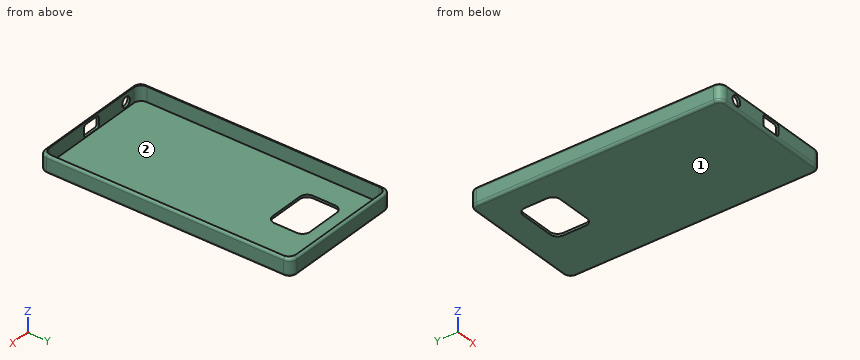
from build123d import *

# Parameters (mm, degrees)
F1_DEPTH = 1
F2_DEPTH = 7
F3_R     = 0.99999
F4_R     = 2
F5_DEPTH = 1


# Not quite as in the source:
# - a fillet or chamfer is up to 0.001 mm smaller than in the source, because OpenCascade refuses the exact size


with BuildPart() as f1:
    # F0 (on Top) → F1 (new body)
    with BuildSketch(Plane.XY):
        with BuildLine():
            Line((26, -48), (26, 48))
            ThreePointArc((26, 48), (25.1213203436, 50.1213203436), (23, 51))
            Line((23, 51), (-23, 51))
            ThreePointArc((-23, 51), (-25.1213203436, 50.1213203436), (-26, 48))
            Line((-26, 48), (-26, -48))
            ThreePointArc((-26, -48), (-25.1213203436, -50.1213203436), (-23, -51))
            Line((-23, -51), (23, -51))
            ThreePointArc((23, -51), (25.1213203436, -50.1213203436), (26, -48))
        make_face()
        with BuildLine():
            ThreePointArc((-25, 47), (-24.1213203436, 49.1213203436), (-22, 50))
            Line((-22, 50), (22, 50))
            ThreePointArc((22, 50), (24.1213203436, 49.1213203436), (25, 47))
            Line((25, 47), (25, -47))
            ThreePointArc((25, -47), (24.1213203436, -49.1213203436), (22, -50))
            Line((22, -50), (-22, -50))
            ThreePointArc((-22, -50), (-24.1213203436, -49.1213203436), (-25, -47))
            Line((-25, -47), (-25, 47))
        make_face(mode=Mode.SUBTRACT)
        with BuildLine():
            Line((22, 50), (-22, 50))
            ThreePointArc((-22, 50), (-24.1213203436, 49.1213203436), (-25, 47))
            Line((-25, 47), (-25, -47))
            ThreePointArc((-25, -47), (-24.1213203436, -49.1213203436), (-22, -50))
            Line((-22, -50), (22, -50))
            ThreePointArc((22, -50), (24.1213203436, -49.1213203436), (25, -47))
            Line((25, -47), (25, 47))
            ThreePointArc((25, 47), (24.1213203436, 49.1213203436), (22, 50))
        make_face()
        with BuildLine():
            ThreePointArc((-15, 37), (-14.1213203436, 39.1213203436), (-12, 40))
            Line((-12, 40), (2, 40))
            ThreePointArc((2, 40), (4.1213203436, 39.1213203436), (5, 37))
            Line((5, 37), (5, 28))
            ThreePointArc((5, 28), (4.1213203436, 25.8786796564), (2, 25))
            Line((2, 25), (-12, 25))
            ThreePointArc((-12, 25), (-14.1213203436, 25.8786796564), (-15, 28))
            Line((-15, 28), (-15, 37))
        make_face(mode=Mode.SUBTRACT)
    extrude(amount=F1_DEPTH)

    # F0 (on Top) → F2 (join)
    with BuildSketch(Plane.XY):
        with BuildLine():
            Line((26, -48), (26, 48))
            ThreePointArc((26, 48), (25.1213203436, 50.1213203436), (23, 51))
            Line((23, 51), (-23, 51))
            ThreePointArc((-23, 51), (-25.1213203436, 50.1213203436), (-26, 48))
            Line((-26, 48), (-26, -48))
            ThreePointArc((-26, -48), (-25.1213203436, -50.1213203436), (-23, -51))
            Line((-23, -51), (23, -51))
            ThreePointArc((23, -51), (25.1213203436, -50.1213203436), (26, -48))
        make_face()
        with BuildLine():
            ThreePointArc((-25, 47), (-24.1213203436, 49.1213203436), (-22, 50))
            Line((-22, 50), (22, 50))
            ThreePointArc((22, 50), (24.1213203436, 49.1213203436), (25, 47))
            Line((25, 47), (25, -47))
            ThreePointArc((25, -47), (24.1213203436, -49.1213203436), (22, -50))
            Line((22, -50), (-22, -50))
            ThreePointArc((-22, -50), (-24.1213203436, -49.1213203436), (-25, -47))
            Line((-25, -47), (-25, 47))
        make_face(mode=Mode.SUBTRACT)
    extrude(amount=F2_DEPTH)

    # F3 (radius 1 in the source; OpenCascade refuses exactly that, so slightly less here)
    f3_edges = [f1.edges().sort_by_distance(p)[0] for p in [
        (26, 0, 0),
        (-26, 0, 7),
    ]]
    fillet(f3_edges, radius=F3_R)

    # F4 (on face) → F5 (cut, through all)
    with BuildSketch(Plane.XZ.offset(51)):
        with BuildLine():
            Line((2.9, 6), (-2.9, 6))
            ThreePointArc((-2.9, 6), (-3.6071067812, 5.7071067812), (-3.9, 5))
            Line((-3.9, 5), (-3.9, 2.2120511904))
            ThreePointArc((-3.9, 2.2120511904), (-3.6071067812, 1.5049444092), (-2.9, 1.2120511904))
            Line((-2.9, 1.2120511904), (2.9, 1.2120511904))
            ThreePointArc((2.9, 1.2120511904), (3.6071067812, 1.5049444092), (3.9, 2.2120511904))
            Line((3.9, 2.2120511904), (3.9, 5))
            ThreePointArc((3.9, 5), (3.6071067812, 5.7071067812), (2.9, 6))
        make_face()
        with Locations((-18, 3.5)):
            Circle(F4_R)
    extrude(amount=-F5_DEPTH, mode=Mode.SUBTRACT)


solid = f1.part
Source: CAD feature listing. Evaluate the final solid. Frame: model axes, mm. Face numbers are marked on the shaded views. Round coordinates to 2 decimals unless told otherwise and drop trailing zeros. Loops run counter-clockwise (first coordinate to the right, second up) from the corner with the lowest first, then second, coordinate; pieces in that order, holes last. Notation, with made-up numbers: M 74.25,23.5 L 109.25,23.5 A23 cw 109.25,61.5 Z; hole C -34.75,76 d5. An arc over 180 degrees is marked long. Answer as CSV lines item,"result".
Q1. Cut plane B-B (z = 3.5). Return the cut outline in (x, y), plus the area to 3 significant figures.
Verdict:
outline,"M -26,-48 A3 ccw -23,-51 L -20,-51 L -20,-50 L -22,-50 A3 cw -25,-47 L -25,47 A3 cw -22,50 L 22,50 A3 cw 25,47 L 25,-47 A3 cw 22,-50 L 3.9,-50 L 3.9,-51 L 23,-51 A3 ccw 26,-48 L 26,48 A3 ccw 23,51 L -23,51 A3 ccw -26,48 Z; M -16,-51 L -3.9,-51 L -3.9,-50 L -16,-50 Z"
area,"292 mm^2"
Q2. Contact query for flat-ended pins moving along their axis: pin 1 (25 mm diameter, centred on x = -4.5, y = 2.5, fed in from +Z); pin 2 (1.8 mm diameter, centred on x = 1.5, z = 3.5, fed in from -Y); pin 3 (0.5 mm diameter, centred on x = 1, y = -50.5, fed in from -Z). Output: stop coordinate, or through.
Verdict:
pin 1,"stops at z = 1"
pin 2,"stops at y = 50"
pin 3,"stops at z = 0.03"
Q3. Line query: line 1 along Y through (x, z) = (-8.5, 2.5); line 2 along X through (y, z) = (-45, 5.5); line 3 along Y through (x, z) = (0.5, 3). Output: solid intervals per line, ascending.
Verdict:
line 1,"y = -51 to -50, 50 to 51"
line 2,"x = -26 to -25, 25 to 26"
line 3,"y = 50 to 51"
Q4. Pull-direction query (X, two-part tool) for the marked faces 1 and 2; classes: +X half, -X half, draft (parallel to the pull), parting line (faces both ways), or undercut.
Verdict:
face 1,"draft"
face 2,"undercut"
Q5. Cut plane D-D (x = 1). Count the separate pieces of the cut face and the enclosed holes in it, plus the area to 3 significant figures.
Verdict:
separate pieces,"3"
enclosed holes,"0"
area,"93.4 mm^2"
